Model file for the job. Use its own axes, mm. Face numbers are marked on the shaded views. A direction names the side the tool comes from. Give positions to 0.01 mm unless a question says otherwise; leave off trailing zeros. Order: outer loops, then holes, each group sorted by start corner. A loop starts at its lowest first (then second) coordinate and runs counter-clockwise, first axis right, second up. Notation, with made-up numbers: (70.5, -1.75) -> (111.5, -1.75) arc R22 ccw to (111.5, 9.25) -> close; hole circle Ø5 at (69.25, 46). An arc over 180 degrees is marked (long way). Answer in a Markdown table with one row per item. Add a question column.
from build123d import *

# Parameters (mm, degrees)
SALIENTE_EXTRUIR1_DEPTH = 80
CROQUIS2_R              = 13
CROQUIS2_R_2            = 4
CROQUIS2_R_3            = 4.5
CORTAR_EXTRUIR1_DEPTH   = 105.637469388
CROQUIS4_R              = 7
CORTAR_EXTRUIR2_DEPTH   = 8.5
CORTAR_EXTRUIR3_REACH   = 106.637
CROQUIS5_R              = 5.5
CROQUIS6_R              = 8.5
CORTAR_EXTRUIR4_DEPTH   = 13
CROQUIS7_R              = 3
CORTAR_EXTRUIR5_DEPTH   = 30


with BuildPart() as part:
    # Croquis1 → Saliente-Extruir1 (new body)
    with BuildSketch(Plane.XY):
        Polygon((65, 0), (-65, 0), (-65, -16), (-45, -16), (-45, -18), (45, -18), (45, -16), (65, -16), align=None)
    extrude(amount=-SALIENTE_EXTRUIR1_DEPTH)

    # Croquis2 → Cortar-Extruir1 (cut, through all)
    with BuildSketch(Plane(origin=(0, 0, 0), x_dir=(1, 0, 0), z_dir=(0, 1, 0))):
        with Locations(Location((0, 40, 0), (0, 0, 180))):
            Circle(CROQUIS2_R)
        with Locations(Location((-55, 70, 0), (0, 0, 180))):
            Circle(CROQUIS2_R_2)
        with Locations(Location((-55, 10, 0), (0, 0, 180))):
            Circle(CROQUIS2_R_2)
        with Locations(Location((55, 10, 0), (0, 0, 180))):
            Circle(CROQUIS2_R_2)
        with Locations(Location((55, 70, 0), (0, 0, 180))):
            Circle(CROQUIS2_R_2)
        with Locations(Location((-55, 58, 0), (0, 0, 180))):
            Circle(CROQUIS2_R_3)
        with Locations(Location((-55, 22, 0), (0, 0, 180))):
            Circle(CROQUIS2_R_3)
        with Locations(Location((55, 58, 0), (0, 0, 180))):
            Circle(CROQUIS2_R_3)
        with Locations(Location((55, 22, 0), (0, 0, 180))):
            Circle(CROQUIS2_R_3)
    extrude(amount=-CORTAR_EXTRUIR1_DEPTH, mode=Mode.SUBTRACT)

    # Croquis4 → Cortar-Extruir2 (cut)
    with BuildSketch(Plane(origin=(0, 0, 0), x_dir=(1, 0, 0), z_dir=(0, 1, 0))):
        with Locations(Location((-55, 58, 0), (0, 0, 180))):
            Circle(CROQUIS4_R)
        with Locations(Location((-55, 22, 0), (0, 0, 180))):
            Circle(CROQUIS4_R)
        with Locations(Location((55, 58, 0), (0, 0, 180))):
            Circle(CROQUIS4_R)
        with Locations(Location((55, 22, 0), (0, 0, 180))):
            Circle(CROQUIS4_R)
    extrude(amount=-CORTAR_EXTRUIR2_DEPTH, mode=Mode.SUBTRACT)

    # Croquis5 → Cortar-Extruir3 (cut, up to next)
    with BuildSketch(Plane(origin=(0, 0, 0), x_dir=(1, 0, 0), z_dir=(0, 1, 0)), mode=Mode.PRIVATE) as cortar_extruir3_sk1:
        with Locations(Location((-25, 65, 0), (0, 0, 180))):
            Circle(CROQUIS5_R)
    cortar_extruir3_tool1 = extrude(cortar_extruir3_sk1.sketch, amount=-CORTAR_EXTRUIR3_REACH, mode=Mode.PRIVATE) & part.part
    # Croquis5 → Cortar-Extruir3 (cut, up to next)
    with BuildSketch(Plane(origin=(0, 0, 0), x_dir=(1, 0, 0), z_dir=(0, 1, 0)), mode=Mode.PRIVATE) as cortar_extruir3_sk2:
        with Locations(Location((-25, 15, 0), (0, 0, 180))):
            Circle(CROQUIS5_R)
    cortar_extruir3_tool2 = extrude(cortar_extruir3_sk2.sketch, amount=-CORTAR_EXTRUIR3_REACH, mode=Mode.PRIVATE) & part.part
    # Croquis5 → Cortar-Extruir3 (cut, up to next)
    with BuildSketch(Plane(origin=(0, 0, 0), x_dir=(1, 0, 0), z_dir=(0, 1, 0)), mode=Mode.PRIVATE) as cortar_extruir3_sk3:
        with Locations(Location((25, 15, 0), (0, 0, 180))):
            Circle(CROQUIS5_R)
    cortar_extruir3_tool3 = extrude(cortar_extruir3_sk3.sketch, amount=-CORTAR_EXTRUIR3_REACH, mode=Mode.PRIVATE) & part.part
    # Croquis5 → Cortar-Extruir3 (cut, up to next)
    with BuildSketch(Plane(origin=(0, 0, 0), x_dir=(1, 0, 0), z_dir=(0, 1, 0)), mode=Mode.PRIVATE) as cortar_extruir3_sk4:
        with Locations(Location((25, 65, 0), (0, 0, 180))):
            Circle(CROQUIS5_R)
    cortar_extruir3_tool4 = extrude(cortar_extruir3_sk4.sketch, amount=-CORTAR_EXTRUIR3_REACH, mode=Mode.PRIVATE) & part.part
    add(cortar_extruir3_tool1.solids().sort_by_distance((-25, 0, -65))[0], mode=Mode.SUBTRACT)
    add(cortar_extruir3_tool2.solids().sort_by_distance((-25, 0, -15))[0], mode=Mode.SUBTRACT)
    add(cortar_extruir3_tool3.solids().sort_by_distance((25, 0, -15))[0], mode=Mode.SUBTRACT)
    add(cortar_extruir3_tool4.solids().sort_by_distance((25, 0, -65))[0], mode=Mode.SUBTRACT)

    # Croquis6 → Cortar-Extruir4 (cut)
    with BuildSketch(Plane(origin=(0, 0, 0), x_dir=(1, 0, 0), z_dir=(0, 1, 0))):
        with Locations(Location((-25, 65, 0), (0, 0, 180))):
            Circle(CROQUIS6_R)
        with Locations(Location((-25, 15, 0), (0, 0, 180))):
            Circle(CROQUIS6_R)
        with Locations(Location((25, 15, 0), (0, 0, 180))):
            Circle(CROQUIS6_R)
        with Locations(Location((25, 65, 0), (0, 0, 180))):
            Circle(CROQUIS6_R)
    extrude(amount=-CORTAR_EXTRUIR4_DEPTH, mode=Mode.SUBTRACT)

    # Croquis7 → Cortar-Extruir5 (cut)
    with BuildSketch(Plane(origin=(0, 0, -80), x_dir=(-1, 0, 0), z_dir=(0, 0, -1))):
        with Locations((38, -8)):
            Circle(CROQUIS7_R)
        with Locations((-38, -8)):
            Circle(CROQUIS7_R)
    extrude(amount=-CORTAR_EXTRUIR5_DEPTH, mode=Mode.SUBTRACT)


solid = part.part
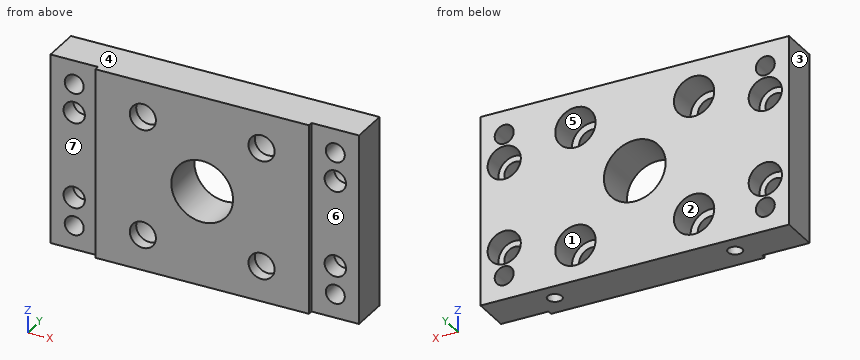
Item 1: Wall check: line 1 (Z direction, x = -25, y = -7); line 2 (Z direction, x = 25, y = -16.75); line 3 (X direction, y = -12.25, z = -56). Give the ranges that are in metal, low to high.
Item 2: Two-plate mould, pull along Z, no slides. Class the marked faces 1, 2, 3 and 4: pulls with the +Z half, pulls with the -Z half, needs draft (parallel to the pull), parting line crosses it, or undercut.
Item 3: Saw through at A-A on x = -55. List the corners of the cut face in (y, z).
Item 4: Saw through at D-D on z = -8. List the corners of the cut face in (x, y), plus the area to 3 significant figures.
Item 5: Which spindle directions (+Z, -Z, +X, -X, +Y, -Y) get a long thin tool onto all of the face, cutting with end or side? Do the marked faces 5, 6 and 7. Say none if no direction does.
Item 6: Saw through at B-B on z = -40. List the corners of the cut face in (x, y), plus the area to 3 significant figures.
Item 7: Saw through at C-C on y = -9.75. Give the number of separate pieces and of enclosed holes in the cut face, plus the area to 3 significant figures.
Item 8: Pin check, flat tips, straight feed: pin 1 Ø15.5 at (x, z) = (-55, -25) entering from +Y; pin 2 Ø13 at (x, z) = (-55, -70) entering from -Y; pin 3 Ø13.5 at (x, z) = (-25, -65) entering from +Y; pin 4 Ø5 at (x, z) = (25.5, -63) entering from +Y. Stop position of each tip, or through.
Evaluation:
| question | item | result |
|---|---|---|
| 1 | line 1 | z = -80 to -73.5, -56.5 to -23.5, -6.5 to 0 |
| 1 | line 2 | z = -80 to -70.5, -59.5 to -20.5, -9.5 to 0 |
| 1 | line 3 | x = -65 to -59.03, -50.97 to 50.97, 59.03 to 65 |
| 2 | face 1 | undercut |
| 2 | face 2 | undercut |
| 2 | face 3 | needs draft |
| 2 | face 4 | pulls with the +Z half |
| 3 | outline | (-16, -80) -> (0, -80) -> (0, -74) -> (-16, -74) -> close; (-16, -66) -> (0, -66) -> (0, -65) -> (-8.5, -65) -> (-8.5, -62.5) -> (-16, -62.5) -> close; (-16, -53.5) -> (-8.5, -53.5) -> (-8.5, -51) -> (0, -51) -> (0, -29) -> (-8.5, -29) -> (-8.5, -26.5) -> (-16, -26.5) -> close; (-16, -17.5) -> (-8.5, -17.5) -> (-8.5, -15) -> (0, -15) -> (0, -14) -> (-16, -14) -> close; (-16, -6) -> (0, -6) -> (0, 0) -> (-16, 0) -> close |
| 4 | outline | (-65, -16) -> (-58.46, -16) -> (-58.46, 0) -> (-65, 0) -> close; (-51.54, -16) -> (-45, -16) -> (-45, -18) -> (45, -18) -> (45, -16) -> (51.54, -16) -> (51.54, 0) -> (29.82, 0) -> (29.82, -13) -> (20.18, -13) -> (20.18, 0) -> (-20.18, 0) -> (-20.18, -13) -> (-29.82, -13) -> (-29.82, 0) -> (-51.54, 0) -> close; (58.46, -16) -> (65, -16) -> (65, 0) -> (58.46, 0) -> close |
| 4 | area | 1,790 mm2 |
| 5 | face 5 | +Y |
| 5 | face 6 | +Z, -Z, +X, -Y |
| 5 | face 7 | +Z, -Z, -X, -Y |
| 6 | outline | (-65, -16) -> (-45, -16) -> (-45, -18) -> (-13, -18) -> (-13, 0) -> (-65, 0) -> close; (13, -18) -> (45, -18) -> (45, -16) -> (65, -16) -> (65, 0) -> (13, 0) -> close |
| 6 | area | 1,790 mm2 |
| 7 | separate pieces | 1 |
| 7 | enclosed holes | 13 |
| 7 | area | 8,210 mm2 |
| 8 | pin 1 | stops at y = 0 |
| 8 | pin 2 | stops at y = -16 |
| 8 | pin 3 | stops at y = -13 |
| 8 | pin 4 | passes through |
